Geometry check sheet. Reference: the model listing, model coordinates, mm. Round coordinates to 2 decimals unless told otherwise and drop trailing zeros. Order: outer loops, then holes, each group sorted by start corner. A loop starts at its lowest first (then second) coordinate and runs counter-clockwise, first axis right, second up. Notation, with made-up numbers: (-17, 6.5) -> (2, 6.5) arc R15 ccw to (2, 11.5) -> close; hole circle Ø9 at (32, 62.25). An arc over 180 degrees is marked (long way). Answer as a JSON object with one key per item and string values. Group by question number.
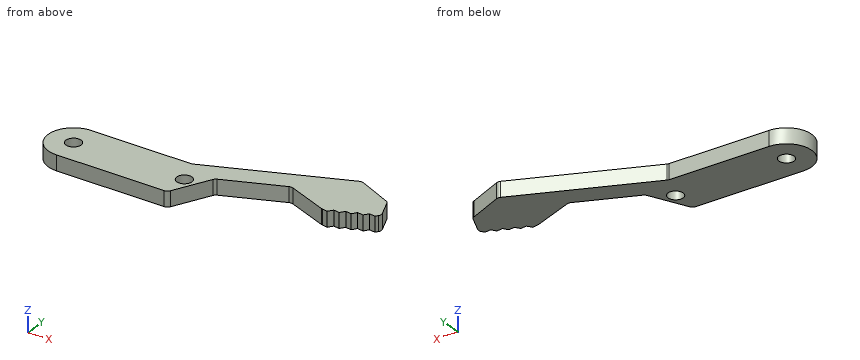
from build123d import *

# Parameters (mm, degrees)
SKETCH_1_R      = 1.5
EXTRUDE_2_DEPTH = 3
FILLET_1_R      = 1
SCALE_1_SCALE   = 2.2


with BuildPart() as part:
    # Эскиз1 → Бобышка-Вытянуть2 (new body)
    with BuildSketch(Plane.XY):
        with BuildLine():
            Line((20.05, 5), (0, 5))
            ThreePointArc((0, 5), (-5, 0), (0, -5))
            Line((0, -5), (22, -5))
            Line((22, -5), (26.028944646, 2.961014192))
            Line((26.028944646, 2.961014192), (37.885430155, 7.835804738))
            Line((37.885430155, 7.835804738), (46.188488025, 4.540007042))
            Line((46.188488025, 4.540007042), (47.351030887, 4.342221563))
            Line((47.351030887, 4.342221563), (48.038244482, 5.300533868))
            Line((48.038244482, 5.300533868), (49.200787343, 5.102748388))
            Line((49.200787343, 5.102748388), (49.888000938, 6.061060693))
            Line((49.888000938, 6.061060693), (51.050543799, 5.863275214))
            Line((51.050543799, 5.863275214), (51.737757394, 6.821587519))
            Line((51.737757394, 6.821587519), (52.900300256, 6.623802039))
            Line((52.900300256, 6.623802039), (53.587513851, 7.582114344))
            Line((53.587513851, 7.582114344), (54.750056712, 7.384328864))
            Line((54.750056712, 7.384328864), (55.437270307, 8.34264117))
            Line((55.437270307, 8.34264117), (53.72608495, 12.504593197))
            Line((53.72608495, 12.504593197), (46.409029503, 15.837507263))
            Line((46.409029503, 15.837507263), (20.05, 5))
        make_face()
        Circle(SKETCH_1_R, mode=Mode.SUBTRACT)
        with Locations((22, 0)):
            Circle(SKETCH_1_R, mode=Mode.SUBTRACT)
    extrude(amount=-EXTRUDE_2_DEPTH)

    # Скругление1
    fillet_1_edges = [part.edges().sort_by_distance(p)[0] for p in [
        (46.188488025, 4.540007042, -1.5),
        (37.885430155, 7.835804738, -1.5),
        (26.028944646, 2.961014192, -1.5),
        (22, -5, -1.5),
        (20.05, 5, -1.5),
        (46.409029503, 15.837507263, -1.5),
        (53.72608495, 12.504593197, -1.5),
        (55.437270307, 8.34264117, -1.5),
    ]]
    fillet(fillet_1_edges, radius=FILLET_1_R)


with BuildPart() as part_1:
    # Масштаб1: scaled about (23.340461949, 3.94478372, -1.5)
    add(part.part.scale(SCALE_1_SCALE).moved(Location((-28.008554339, -4.733740464, 1.8))))


solid = part_1.part
Item 1: Sectioned sample at B-B, the plane x = 6. Enter the section's corners in (y, z).
Item 2: Sectioned sample at C-C, the plane y = 27.5. Enter the section's corners in (x, z), then the cut area to 3 significant figures.
Item 3: Thickness scan on L1, parallel to X at y = -3, z = -2.5; L2, parallel to X at y = -3.5, z = 1.25; L3, parallel to Y at x = -16.5, z = -4.25. Record the ranges inside material, lowest first.
Item 4: Sectioned sample at A-A, the plane z = -3.5. Count the separate pieces of the cut face and the enclosed holes in it, then the cut area to 3 significant figures.
Item 5: Depth check by flat-ended pin: pin 1 Ø8.5 at (x, y) = (20.39, -4.73) entering from +Z; pin 2 Ø1.5 at (x, z) = (-10, -3) entering from +Y; pin 3 Ø5.5 at (x, y) = (-28.01, -4.73) entering from -Z. Enter the tip coordinate at first touch or a pass-through.
Result:
{
 "1": {"outline": "(-15.73, -4.8) -> (6.27, -4.8) -> (6.27, 1.8) -> (-15.73, 1.8) -> close"},
 "2": {"outline": "(67.75, -4.8) -> (79.82, -4.8) -> (79.82, 1.8) -> (67.75, 1.8) -> close", "area": "79.7 mm2"},
 "3": {"L1": "x = -38.87 to -30.82, -25.2 to 17.58, 23.2 to 26.84", "L2": "x = -38.94 to -31.07, -24.95 to 17.33, 23.45 to 26.58", "L3": "y = -15.73 to 6.27"},
 "4": {"separate pieces": "1", "enclosed holes": "2", "area": "2,240 mm2"},
 "5": {"pin 1": "stops at z = 1.8", "pin 2": "stops at y = 6.27", "pin 3": "passes through"}
}
